```python
from build123d import *

# Parameters (mm, degrees)
F0_R     = 150
F0_R_2   = 100
F1_DEPTH = 200
F2_SIZE  = 20
F3_SIZE  = 20
F4_SIZE  = 5.08
F5_SIZE  = 5.08


with BuildPart() as f1:
    # F0 (on Right) → F1 (new body)
    with BuildSketch(Plane.YZ):
        Circle(F0_R)
        Circle(F0_R_2, mode=Mode.SUBTRACT)
    extrude(amount=F1_DEPTH)

    # F2
    f2_edges = [f1.edges().sort_by_distance(p)[0] for p in [
        (200, -150, 0),
    ]]
    chamfer(f2_edges, length=F2_SIZE)

    # F3
    f3_edges = [f1.edges().sort_by_distance(p)[0] for p in [
        (0, -150, 0),
    ]]
    chamfer(f3_edges, length=F3_SIZE)

    # F4
    f4_edges = [f1.edges().sort_by_distance(p)[0] for p in [
        (200, -100, 0),
    ]]
    chamfer(f4_edges, length=F4_SIZE)

    # F5
    f5_edges = [f1.edges().sort_by_distance(p)[0] for p in [
        (0, -100, 0),
    ]]
    chamfer(f5_edges, length=F5_SIZE)


solid = f1.part
```
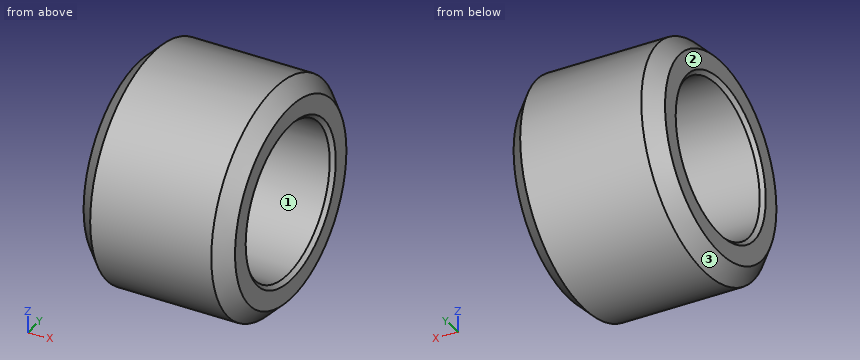
Work out the finished part from the listing and answer in its coordinate system (mm). Face numbers are marked on the shaded views. Give positions to 0.01 mm unless a question says otherwise; leave off trailing zeros. Loops run counter-clockwise (first coordinate to the right, second up) from the corner with the lowest first, then second, coordinate; pieces in that order, holes last. Notation, with made-up numbers: M 76.25,61 L 85.25,61 A22 cw 85.25,80 Z; hole C 58.5,-17.75 d2. An arc over 180 degrees is marked long. One line per item, written item: value. Start each with the question number.
1. Each of these flat-tipped pins is pushed along its axis until it touches: P1, Ø10, axis at x = 81, z = 43.5, coming from the -Y side (3 decimals); P2, Ø6, axis at x = 147, y = -52.5, coming from the -Z side; P3, Ø1, axis at x = 60.5, y = -76, coming from the -Z side. Where does it stop, or does it pass through?
2. Find section D-D (x = 13). Give the vertices of the cut face in (y, z), and give its area (3 significant figures).
3. Determine the mould class of the marked faces 1, 2 and 3 for opening direction Y: released by +Y, released by -Y, zero draft, split by the parting line, or undercut.
4. Find the intervals of material crossed by probe 1 along Z at (x, y) = (104, 0); probe 2 along Z at (x, y) = (145, 76); probe 3 along Y at (x, z) = (30.5, 5.5), in increasing order.
5. Find section C-C (x = 151). Give the vertices of the cut face in (y, z).
6. Find section A-A (z = 0). Give the vertices of the cut face in (x, y).
Reported:
1. P1: stops at y = -144.975
1. P2: stops at z = -141.6
1. P3: stops at z = -129.61
2. outline: C 0,0 d286; hole C 0,0 d200
2. area: 32,800 mm²
3. face 1: undercut
3. face 2: zero draft
3. face 3: split by the parting line
4. probe 1: z = -150 to -100, 100 to 150
4. probe 2: z = -129.32 to -64.99, 64.99 to 129.32
4. probe 3: y = -149.9 to -99.85, 99.85 to 149.9
5. outline: C 0,0 d300; hole C 0,0 d200
6. outline: M 0,-130 L 20,-150 L 180,-150 L 200,-130 L 200,-105.08 L 194.92,-100 L 5.08,-100 L 0,-105.08 Z; M 0,105.08 L 5.08,100 L 194.92,100 L 200,105.08 L 200,130 L 180,150 L 20,150 L 0,130 Z
